```python
from build123d import *

# Parameters (mm, degrees)
BOSS_EXTRUDE2_DEPTH     = 25.654
BOSS_EXTRUDE4_DEPTH     = 3.175
BOSS_EXTRUDE5_DEPTH     = 16.141204421
CUT_EXTRUDE1_DEPTH      = 36.068
CUT_EXTRUDE1_DEPTH_BACK = 99.314
SKETCH8_W               = 5.954134369
SKETCH8_H               = 7.391339216
SKETCH8_3_W             = 5.954134368
SKETCH8_3_H             = 7.391339216
SKETCH8_3_W_2           = 5.954134369
CUT_EXTRUDE2_DEPTH      = 99.314
SKETCH10_W              = 114.3
SKETCH10_H              = 87.072843295
BOSS_EXTRUDE7_DEPTH     = 3.81
SKETCH11_W              = 12.814534476
SKETCH11_H              = 54.915455345
CUT_EXTRUDE4_DEPTH      = 23.368
SKETCH18_W              = 3.81
SKETCH18_H              = 39.122149616
BOSS_EXTRUDE10_DEPTH    = 10.16
CUT_EXTRUDE5_DEPTH      = 33.528
CUT_EXTRUDE5_DEPTH_BACK = 93.218
SKETCH20_R              = 2.0193
CUT_EXTRUDE7_REACH      = 108.861
SKETCH21_R              = 1.375
FILLET1_R               = 2.54
FILLET2_R               = 2.54
FILLET3_R               = 2.54
FILLET4_R               = 5.08


with BuildPart() as part:
    # Sketch1 → Boss-Extrude2 (new body)
    with BuildSketch(Plane(origin=(0, 0, 0), x_dir=(1, 0, 0), z_dir=(0, 1, 0))):
        Polygon((26.716415821, 45.081669174), (26.716415821, -39.405390864), (29.891415821, -39.405390864), (29.891415821, 47.667452431), (-84.408584179, 47.667452431), (-84.408584179, -39.405390864), (-81.233584179, -39.405390864), (-81.233584179, 45.081669174), align=None)
    extrude(amount=BOSS_EXTRUDE2_DEPTH)

    # Sketch3 → Boss-Extrude4 (add)
    with BuildSketch(Plane(origin=(0, 25.654, 0), x_dir=(1, 0, 0), z_dir=(0, 1, 0))):
        Polygon((4.379625861, -39.405390864), (26.716415821, -39.405390864), (29.891415821, -39.405390864), (29.891415821, 47.667452431), (26.716415821, 47.667452431), (26.716415821, 45.081669174), (4.379625861, 45.081669174), (4.379625861, -0.014587754), align=None)
        Polygon((-60.331822089, 45.081669174), (4.379625861, 45.081669174), (26.716415821, 45.081669174), (26.716415821, 47.667452431), (-81.233584179, 47.667452431), (-84.408584179, 47.667452431), (-84.408584179, -39.405390864), (-78.531426376, -39.405390864), (-60.331822089, -39.405390864), (-60.331822089, -0.014587754), align=None)
    extrude(amount=BOSS_EXTRUDE4_DEPTH)

    # Sketch4 → Boss-Extrude5 (add)
    with BuildSketch(Plane(origin=(0, 28.829, 0), x_dir=(1, 0, 0), z_dir=(0, 1, 0))):
        Polygon((-64.141822089, -0.283241248), (-60.331822089, -0.283241248), (-60.331822089, 45.081669174), (4.379625861, 45.081669174), (4.379625861, -0.283241248), (8.189625861, -0.283241248), (8.189625861, 47.667452431), (-64.141822089, 47.667452431), align=None)
    extrude(amount=BOSS_EXTRUDE5_DEPTH)

    # Sketch8 → Cut-Extrude1 (cut, two sides: drawn at the far end of the back side and taken through both)
    with BuildSketch(Plane(origin=(8.189625861, 0, 0), x_dir=(0, 0, -1), z_dir=(1, 0, 0)).offset(-CUT_EXTRUDE1_DEPTH_BACK)):
        with Locations((18.262175985, 35.424269821)):
            Rectangle(SKETCH8_W, SKETCH8_H)
    extrude(amount=CUT_EXTRUDE1_DEPTH + CUT_EXTRUDE1_DEPTH_BACK, mode=Mode.SUBTRACT)

    # Sketch8_3 → Cut-Extrude2 (cut)
    with BuildSketch(Plane(origin=(8.189625861, 0, 0), x_dir=(0, 0, -1), z_dir=(1, 0, 0))):
        with Locations((41.087726864, 35.434837043)):
            Rectangle(SKETCH8_3_W, SKETCH8_3_H)
        with Locations((29.674951425, 35.429553432)):
            Rectangle(SKETCH8_3_W_2, SKETCH8_3_H)
        with Locations((18.262175985, 35.424269821)):
            Rectangle(SKETCH8_3_W_2, SKETCH8_3_H)
        with Locations((6.849400545, 35.41898621)):
            Rectangle(SKETCH8_3_W, SKETCH8_3_H)
    extrude(amount=-CUT_EXTRUDE2_DEPTH, mode=Mode.SUBTRACT)

    # Sketch10 → Boss-Extrude7 (add)
    with BuildSketch(Plane(origin=(0, 0, 0), x_dir=(1, 0, 0), z_dir=(0, 1, 0))):
        with Locations((-27.258584179, 4.131030783)):
            Rectangle(SKETCH10_W, SKETCH10_H)
    extrude(amount=-BOSS_EXTRUDE7_DEPTH)

    # Sketch11 → Cut-Extrude4 (cut)
    with BuildSketch(Plane(origin=(0, 6.655, 0), x_dir=(1, 0, 0), z_dir=(0, 1, 0))):
        with Locations((16.472358623, 9.22876842)):
            Rectangle(SKETCH11_W, SKETCH11_H)
    extrude(amount=CUT_EXTRUDE4_DEPTH, mode=Mode.SUBTRACT)

    # Sketch18 → Boss-Extrude10 (add)
    with BuildSketch(Plane(origin=(0, 28.829, 0), x_dir=(1, 0, 0), z_dir=(0, 1, 0))):
        with Locations((-62.236822089, -19.844316056)):
            Rectangle(SKETCH18_W, SKETCH18_H)
        with Locations((6.284625861, -19.844316056)):
            Rectangle(SKETCH18_W, SKETCH18_H)
    extrude(amount=BOSS_EXTRUDE10_DEPTH)

    # Sketch20 → Cut-Extrude5 (cut, two sides: drawn at the far end of the back side and taken through both)
    with BuildSketch(Plane(origin=(8.189625861, 0, 0), x_dir=(0, 0, -1), z_dir=(1, 0, 0)).offset(-CUT_EXTRUDE5_DEPTH_BACK)):
        with Locations(Location((-19.844316056, 33.125886584, 0), (0, 0, 180))):
            Circle(SKETCH20_R)
    extrude(amount=CUT_EXTRUDE5_DEPTH + CUT_EXTRUDE5_DEPTH_BACK, mode=Mode.SUBTRACT)

    # Sketch21 → Cut-Extrude7 (cut, up to next)
    with BuildSketch(Plane(origin=(0, 0, 0), x_dir=(1, 0, 0), z_dir=(0, 1, 0)), mode=Mode.PRIVATE) as cut_extrude7_sk1:
        with Locations(Location((-73.120374139, 39.635412246, 0), (0, 0, 270))):
            Circle(SKETCH21_R)
    cut_extrude7_tool1 = extrude(cut_extrude7_sk1.sketch, amount=-CUT_EXTRUDE7_REACH, mode=Mode.PRIVATE) & part.part
    # Sketch21 → Cut-Extrude7 (cut, up to next)
    with BuildSketch(Plane(origin=(0, 0, 0), x_dir=(1, 0, 0), z_dir=(0, 1, 0)), mode=Mode.PRIVATE) as cut_extrude7_sk2:
        with Locations(Location((12.879625861, 39.635412246, 0), (0, 0, 270))):
            Circle(SKETCH21_R)
    cut_extrude7_tool2 = extrude(cut_extrude7_sk2.sketch, amount=-CUT_EXTRUDE7_REACH, mode=Mode.PRIVATE) & part.part
    # Sketch21 → Cut-Extrude7 (cut, up to next)
    with BuildSketch(Plane(origin=(0, 0, 0), x_dir=(1, 0, 0), z_dir=(0, 1, 0)), mode=Mode.PRIVATE) as cut_extrude7_sk3:
        with Locations(Location((12.879625861, -18.364587754, 0), (0, 0, 270))):
            Circle(SKETCH21_R)
    cut_extrude7_tool3 = extrude(cut_extrude7_sk3.sketch, amount=-CUT_EXTRUDE7_REACH, mode=Mode.PRIVATE) & part.part
    # Sketch21 → Cut-Extrude7 (cut, up to next)
    with BuildSketch(Plane(origin=(0, 0, 0), x_dir=(1, 0, 0), z_dir=(0, 1, 0)), mode=Mode.PRIVATE) as cut_extrude7_sk4:
        with Locations(Location((-73.120374139, -18.364587754, 0), (0, 0, 270))):
            Circle(SKETCH21_R)
    cut_extrude7_tool4 = extrude(cut_extrude7_sk4.sketch, amount=-CUT_EXTRUDE7_REACH, mode=Mode.PRIVATE) & part.part
    add(cut_extrude7_tool1.solids().sort_by_distance((-73.120374, 0, -39.635412))[0], mode=Mode.SUBTRACT)
    add(cut_extrude7_tool2.solids().sort_by_distance((12.879626, 0, -39.635412))[0], mode=Mode.SUBTRACT)
    add(cut_extrude7_tool3.solids().sort_by_distance((12.879626, 0, 18.364588))[0], mode=Mode.SUBTRACT)
    add(cut_extrude7_tool4.solids().sort_by_distance((-73.120374, 0, 18.364588))[0], mode=Mode.SUBTRACT)

    # Fillet1
    fillet1_edges = [part.edges().sort_by_distance(p)[0] for p in [
        (-84.408584179, 12.5095, -47.667452431),
        (29.891415821, 12.5095, -47.667452431),
        (-84.408584179, -3.81, -4.131030784),
        (-27.258584179, -3.81, -47.667452431),
        (29.891415821, -3.81, -4.131030784),
        (29.891415821, 28.829, -4.131030784),
        (19.040520841, 28.829, -47.667452431),
        (-84.408584179, 28.829, -4.131030784),
        (-74.275203134, 28.829, -47.667452431),
    ]]
    fillet(fillet1_edges, radius=FILLET1_R)

    # Fillet2
    fillet2_edges = [part.edges().sort_by_distance(p)[0] for p in [
        (-62.236822089, 39.130506651, -38.11065968),
        (6.284625861, 39.130506651, -38.11065968),
        (-62.236822089, 39.130506651, -44.064794048),
        (6.284625861, 39.130506651, -44.064794048),
        (-62.236822089, 31.739167435, -44.064794048),
        (6.284625861, 31.739167435, -44.064794048),
        (-62.236822089, 31.739167435, -38.11065968),
        (6.284625861, 31.739167435, -38.11065968),
        (-62.236822089, 39.12522304, -32.652018609),
        (6.284625861, 39.12522304, -32.652018609),
        (-62.236822089, 31.733883824, -32.652018609),
        (6.284625861, 31.733883824, -32.652018609),
        (-62.236822089, 31.733883824, -26.69788424),
        (6.284625861, 31.733883824, -26.69788424),
        (-62.236822089, 39.12522304, -26.69788424),
        (6.284625861, 39.12522304, -26.69788424),
        (-62.236822089, 39.114655818, -9.826467729),
        (6.284625861, 39.114655818, -9.826467729),
        (-62.236822089, 31.723316602, -9.826467729),
        (6.284625861, 31.723316602, -9.826467729),
        (-62.236822089, 31.723316602, -3.872333361),
        (6.284625861, 31.723316602, -3.872333361),
        (-62.236822089, 39.114655818, -3.872333361),
        (6.284625861, 39.114655818, -3.872333361),
        (-62.236822089, 39.119939429, -15.2851088),
        (6.284625861, 39.119939429, -15.2851088),
        (-62.236822089, 31.728600213, -15.2851088),
        (6.284625861, 31.728600213, -15.2851088),
        (-62.236822089, 31.728600213, -21.239243169),
        (6.284625861, 31.728600213, -21.239243169),
        (-62.236822089, 39.119939429, -21.239243169),
        (6.284625861, 39.119939429, -21.239243169),
    ]]
    fillet(fillet2_edges, radius=FILLET2_R)

    # Fillet3
    fillet3_edges = [part.edges().sort_by_distance(p)[0] for p in [
        (6.284625861, 38.989, 0.283241248),
        (-62.236822089, 38.989, 0.283241248),
    ]]
    fillet(fillet3_edges, radius=FILLET3_R)

    # Fillet4
    fillet4_edges = [part.edges().sort_by_distance(p)[0] for p in [
        (10.065091385, 27.2415, 18.228959253),
        (22.879625861, 27.2415, 18.228959253),
    ]]
    fillet(fillet4_edges, radius=FILLET4_R)


solid = part.part
```
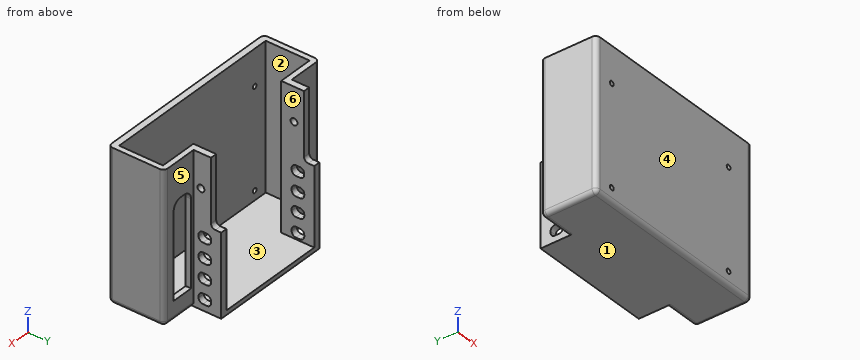
Input: part model. Units: mm. Frame: model coordinates. Face numbers are marked on the shaded views. A direction names the side the tool comes from. Round coordinates to 2 decimals unless told otherwise and drop trailing zeros. Loops run counter-clockwise (first coordinate to the right, second up) from the corner with the lowest first, then second, coordinate; pieces in that order, holes last. Notation, with made-up numbers: (-10, 8) - (41, 8) arc R20 cw to (41, 44) - close; hole circle Ø2 at (-30, -39.5). An arc over 180 degrees is marked (long way). One line per item, written item: value. Start each with the question number.
(1) Access query for the marked faces 1 and 2. Directions: +Z, -Z, +X, -X, +Y, -Y. A direction counts if a zero-diameter tool reaches every point of the face in a straight line with its end or side. Return the directions, or none.
(2) Contact query for flat-ended pins moving along their axis: P1, Ø1.7, axis at x = 7, y = 43.5, coming from the +Z side; P2, Ø2, axis at x = 12.88, z = -39.64, coming from the -Y side; P3, Ø6, axis at x = -33.5, z = -19.5, coming from the +Y side; P4, Ø3, axis at y = 33.13, z = 19.84, coming from the +X side. Output: stop coordinate, or through.
(3) Section B-B, the plane y = 17.5. Return loops of the section in (x, z).
(4) Section C-C, the plane x = -50. Return loops of the section in (y, z).
(5) Section A-A, the plane z = -13.5. Return loops of the section in (x, y).
(6) Ray query, line 1 (X direction, y = 24.5, z = 0.5); line 2 (X direction, y = 27, z = -6); line 3 (Y direction, x = -65.5, z = -42.5). Return the intervals inside material, ascending. Write a range as [from, to].
(7) Draft query along Y for the marked faces 3, 4, 5 and 6. Return one class per face: +Y half, -Y half, draft (parallel to the pull), parting line (faces both ways), or undercut.
Results below:
1. face 1: -Z, +X, -X, +Y, -Y
1. face 2: +Z
2. P1: z = 0.28
2. P2: y = 25.65
2. P3: y = 0
2. P4: through
3. outline: (-84.41, -45.13) arc R2.54 ccw to (-81.87, -47.67) - (27.35, -47.67) arc R2.54 ccw to (29.89, -45.13) - (29.89, 39.41) - (26.72, 39.41) - (26.72, -45.08) - (-81.23, -45.08) - (-81.23, 39.41) - (-84.41, 39.41) - close
4. outline: (-3.81, -45.13) arc R2.54 ccw to (-1.27, -47.67) - (44.97, -47.67) - (44.97, -45.08) - (0, -45.08) - (0, 39.41) - (-3.81, 39.41) - close
5. outline: (-84.41, -1.27) arc R2.54 ccw to (-81.87, -3.81) - (27.35, -3.81) arc R2.54 ccw to (29.89, -1.27) - (29.89, 26.29) arc R2.54 ccw to (27.35, 28.83) - (22.88, 28.83) - (22.88, 25.65) - (26.72, 25.65) - (26.72, 0) - (-81.23, 0) - (-81.23, 25.65) - (-60.33, 25.65) - (-60.33, 44.97) - (-64.14, 44.97) - (-64.14, 28.83) - (-81.87, 28.83) arc R2.54 ccw to (-84.41, 26.29) - close; (4.38, 25.65) - (10.07, 25.65) - (10.07, 28.83) - (8.19, 28.83) - (8.19, 44.97) - (4.38, 44.97) - close
6. line 1: [-84.41, -81.23], [26.72, 29.89]
6. line 2: [-84.31, -60.33], [4.38, 10.07], [22.88, 29.79]
6. line 3: [-3.81, 0], [25.65, 28.83]
7. face 3: undercut
7. face 4: -Y half
7. face 5: +Y half
7. face 6: draft
